from build123d import *

# Parameters (mm, degrees)
SZKIC1_R                    = 3.4
DODANIE_WYCI_GNI_CIE1_DEPTH = 1400


with BuildPart() as part:
    # Szkic1 → Dodanie-wyciągnięcie1 (new body)
    with BuildSketch(Plane.XY):
        with BuildLine():
            Line((-40, -19), (-40, 19))
            ThreePointArc((-40, 19), (-39.707106781, 19.707106781), (-39, 20))
            Line((-39, 20), (-24, 20))
            Line((-24, 20), (-24, 15.5))
            Line((-24, 15.5), (-26.471381771, 15.5))
            Line((-26.471381771, 15.5), (-26.471381771, 17.75))
            ThreePointArc((-26.471381771, 17.75), (-28.062372029, 17.090990258), (-28.721381771, 15.5))
            ThreePointArc((-28.721381771, 15.5), (-27.448087912, 10.962546258), (-24, 7.75))
            Line((-24, 7.75), (-16, 7.75))
            ThreePointArc((-16, 7.75), (-12.551912088, 10.962546258), (-11.278618229, 15.5))
            ThreePointArc((-11.278618229, 15.5), (-11.937627971, 17.090990258), (-13.528618229, 17.75))
            Line((-13.528618229, 17.75), (-13.528618229, 15.5))
            Line((-13.528618229, 15.5), (-16, 15.5))
            Line((-16, 15.5), (-16, 20))
            Line((-16, 20), (13.528618229, 20))
            Line((13.528618229, 20), (16, 20))
            Line((16, 20), (16, 15.5))
            Line((16, 15.5), (13.528618229, 15.5))
            Line((13.528618229, 15.5), (13.528618229, 17.75))
            ThreePointArc((13.528618229, 17.75), (11.937627971, 17.090990258), (11.278618229, 15.5))
            ThreePointArc((11.278618229, 15.5), (12.551912088, 10.962546258), (16, 7.75))
            Line((16, 7.75), (24, 7.75))
            ThreePointArc((24, 7.75), (27.448087912, 10.962546258), (28.721381771, 15.5))
            ThreePointArc((28.721381771, 15.5), (28.062372029, 17.090990258), (26.471381771, 17.75))
            Line((26.471381771, 17.75), (26.471381771, 15.5))
            Line((26.471381771, 15.5), (24, 15.5))
            Line((24, 15.5), (24, 20))
            Line((24, 20), (39, 20))
            ThreePointArc((39, 20), (39.707106781, 19.707106781), (40, 19))
            Line((40, 19), (40, 4))
            Line((40, 4), (35.5, 4))
            Line((35.5, 4), (35.5, 6.471381771))
            Line((35.5, 6.471381771), (37.75, 6.471381771))
            ThreePointArc((37.75, 6.471381771), (37.090990258, 8.062372029), (35.5, 8.721381771))
            ThreePointArc((35.5, 8.721381771), (30.962546258, 7.448087912), (27.75, 4))
            Line((27.75, 4), (27.75, -4))
            ThreePointArc((27.75, -4), (30.962546258, -7.448087912), (35.5, -8.721381771))
            ThreePointArc((35.5, -8.721381771), (37.090990258, -8.062372029), (37.75, -6.471381771))
            Line((37.75, -6.471381771), (35.5, -6.471381771))
            Line((35.5, -6.471381771), (35.5, -4))
            Line((35.5, -4), (40, -4))
            Line((40, -4), (40, -19))
            ThreePointArc((40, -19), (39.707106781, -19.707106781), (39, -20))
            Line((39, -20), (24, -20))
            Line((24, -20), (24, -15.5))
            Line((24, -15.5), (26.471381771, -15.5))
            Line((26.471381771, -15.5), (26.471381771, -17.75))
            ThreePointArc((26.471381771, -17.75), (28.062372029, -17.090990258), (28.721381771, -15.5))
            ThreePointArc((28.721381771, -15.5), (27.448087912, -10.962546258), (24, -7.75))
            Line((24, -7.75), (16, -7.75))
            ThreePointArc((16, -7.75), (12.551912088, -10.962546258), (11.278618229, -15.5))
            ThreePointArc((11.278618229, -15.5), (11.937627971, -17.090990258), (13.528618229, -17.75))
            Line((13.528618229, -17.75), (13.528618229, -15.5))
            Line((13.528618229, -15.5), (16, -15.5))
            Line((16, -15.5), (16, -20))
            Line((16, -20), (-16, -20))
            Line((-16, -20), (-16, -15.5))
            Line((-16, -15.5), (-13.528618229, -15.5))
            Line((-13.528618229, -15.5), (-13.528618229, -17.75))
            ThreePointArc((-13.528618229, -17.75), (-11.937627971, -17.090990258), (-11.278618229, -15.5))
            ThreePointArc((-11.278618229, -15.5), (-12.551912088, -10.962546258), (-16, -7.75))
            Line((-16, -7.75), (-24, -7.75))
            ThreePointArc((-24, -7.75), (-27.448087912, -10.962546258), (-28.721381771, -15.5))
            ThreePointArc((-28.721381771, -15.5), (-28.062372029, -17.090990258), (-26.471381771, -17.75))
            Line((-26.471381771, -17.75), (-26.471381771, -15.5))
            Line((-26.471381771, -15.5), (-24, -15.5))
            Line((-24, -15.5), (-24, -20))
            Line((-24, -20), (-39, -20))
            ThreePointArc((-39, -20), (-39.707106781, -19.707106781), (-40, -19))
        make_face()
        with Locations((-20, 0)):
            Circle(SZKIC1_R, mode=Mode.SUBTRACT)
        with Locations((20, 0)):
            Circle(SZKIC1_R, mode=Mode.SUBTRACT)
        with BuildLine():
            Line((30.971381771, -17.75), (36.75, -17.75))
            ThreePointArc((36.75, -17.75), (37.457106781, -17.457106781), (37.75, -16.75))
            Line((37.75, -16.75), (37.75, -10.971381771))
            Line((37.75, -10.971381771), (30.971381771, -10.971381771))
            Line((30.971381771, -10.971381771), (30.971381771, -17.75))
        make_face(mode=Mode.SUBTRACT)
        with BuildLine():
            Line((-35.5, -6.471381771), (-37.75, -6.471381771))
            ThreePointArc((-37.75, -6.471381771), (-37.090990258, -8.062372029), (-35.5, -8.721381771))
            ThreePointArc((-35.5, -8.721381771), (-30.962546258, -7.448087912), (-27.75, -4))
            Line((-27.75, -4), (-27.75, 4))
            ThreePointArc((-27.75, 4), (-30.962546258, 7.448087912), (-35.5, 8.721381771))
            ThreePointArc((-35.5, 8.721381771), (-37.090990258, 8.062372029), (-37.75, 6.471381771))
            Line((-37.75, 6.471381771), (-35.5, 6.471381771))
            Line((-35.5, 6.471381771), (-35.5, 4))
            Line((-35.5, 4), (-37.75, 4))
            Line((-37.75, 4), (-37.75, -4))
            Line((-37.75, -4), (-35.5, -4))
            Line((-35.5, -4), (-35.5, -6.471381771))
        make_face(mode=Mode.SUBTRACT)
        with BuildLine():
            Line((10.528618229, 7.090188806), (11.40950808, 7.090188806))
            ThreePointArc((11.40950808, 7.090188806), (12.470168251, 6.650848977), (12.90950808, 5.590188806))
            Line((12.90950808, 5.590188806), (12.90950808, -5.590188806))
            ThreePointArc((12.90950808, -5.590188806), (12.470168251, -6.650848977), (11.40950808, -7.090188806))
            Line((11.40950808, -7.090188806), (10.528618229, -7.090188806))
            ThreePointArc((10.528618229, -7.090188806), (9.467958057, -7.529528634), (9.028618229, -8.590188806))
            Line((9.028618229, -8.590188806), (9.028618229, -16.25))
            ThreePointArc((9.028618229, -16.25), (8.589278401, -17.310660172), (7.528618229, -17.75))
            Line((7.528618229, -17.75), (-7.528618229, -17.75))
            ThreePointArc((-7.528618229, -17.75), (-8.589278401, -17.310660172), (-9.028618229, -16.25))
            Line((-9.028618229, -16.25), (-9.028618229, -8.590188806))
            ThreePointArc((-9.028618229, -8.590188806), (-9.467958057, -7.529528634), (-10.528618229, -7.090188806))
            Line((-10.528618229, -7.090188806), (-11.40950808, -7.090188806))
            ThreePointArc((-11.40950808, -7.090188806), (-12.470168251, -6.650848977), (-12.90950808, -5.590188806))
            Line((-12.90950808, -5.590188806), (-12.90950808, 5.590188806))
            ThreePointArc((-12.90950808, 5.590188806), (-12.470168251, 6.650848977), (-11.40950808, 7.090188806))
            Line((-11.40950808, 7.090188806), (-10.528618229, 7.090188806))
            ThreePointArc((-10.528618229, 7.090188806), (-9.467958057, 7.529528634), (-9.028618229, 8.590188806))
            Line((-9.028618229, 8.590188806), (-9.028618229, 16.25))
            ThreePointArc((-9.028618229, 16.25), (-8.589278401, 17.310660172), (-7.528618229, 17.75))
            Line((-7.528618229, 17.75), (7.528618229, 17.75))
            ThreePointArc((7.528618229, 17.75), (8.589278401, 17.310660172), (9.028618229, 16.25))
            Line((9.028618229, 16.25), (9.028618229, 8.590188806))
            ThreePointArc((9.028618229, 8.590188806), (9.467958057, 7.529528634), (10.528618229, 7.090188806))
        make_face(mode=Mode.SUBTRACT)
        with BuildLine():
            Line((30.971381771, 10.971381771), (37.75, 10.971381771))
            Line((37.75, 10.971381771), (37.75, 16.75))
            ThreePointArc((37.75, 16.75), (37.457106781, 17.457106781), (36.75, 17.75))
            Line((36.75, 17.75), (30.971381771, 17.75))
            Line((30.971381771, 17.75), (30.971381771, 10.971381771))
        make_face(mode=Mode.SUBTRACT)
        with BuildLine():
            Line((-30.971381771, -10.971381771), (-30.971381771, -17.75))
            Line((-30.971381771, -17.75), (-36.75, -17.75))
            ThreePointArc((-36.75, -17.75), (-37.457106781, -17.457106781), (-37.75, -16.75))
            Line((-37.75, -16.75), (-37.75, -10.971381771))
            Line((-37.75, -10.971381771), (-30.971381771, -10.971381771))
        make_face(mode=Mode.SUBTRACT)
        with BuildLine():
            Line((-30.971381771, 17.75), (-36.75, 17.75))
            ThreePointArc((-36.75, 17.75), (-37.457106781, 17.457106781), (-37.75, 16.75))
            Line((-37.75, 16.75), (-37.75, 10.971381771))
            Line((-37.75, 10.971381771), (-30.971381771, 10.971381771))
            Line((-30.971381771, 10.971381771), (-30.971381771, 17.75))
        make_face(mode=Mode.SUBTRACT)
    extrude(amount=DODANIE_WYCI_GNI_CIE1_DEPTH)


solid = part.part
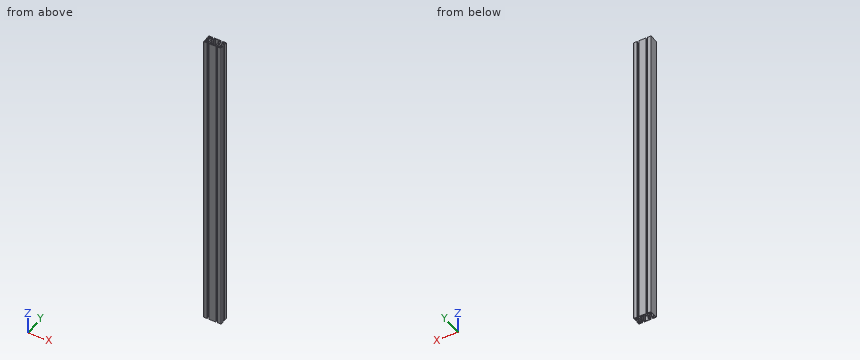
Work out the finished part from the listing and answer in its coordinate system (mm). Round coordinates to 2 decimals unless told otherwise and drop trailing zeros.
1) A cutting plane is placed at A-A (z = 617.5). Give the number of separate pieces and of enclosed holes in the cut face, plus the area to 3 significant figures.
2) Given pin 1 Ø12.5 at (y, z) = (0, 732.5) entering from +X; pin 2 Ø4 at (x, z) = (-21, 427) entering from +Y, each flat-ended and moving along its own axis, determine where each tip first touches the part or whether it passes through.
3) Straight lines are drawn through the part: line 1 (X direction, y = 1, z = 196); line 2 (X direction, y = -15, z = 1332.5); line 3 (Y direction, x = 20, z = 890). For each, find the intervals that lie inside material, in ascending order.
Completed:
1. separate pieces: 1
1. enclosed holes: 8
1. area: 1,260 mm2
2. pin 1: stops at x = 40
2. pin 2: stops at y = 7.75
3. line 1: x = -40 to -37.75, -27.75 to -23.25, -16.75 to -12.91, 12.91 to 16.75, 23.25 to 27.75
3. line 2: x = -40 to -37.75, -30.97 to -28.71, -11.29 to -9.03, 9.03 to 11.29, 28.71 to 30.97, 37.75 to 40
3. line 3: y = -7.75 to -3.4, 3.4 to 7.75
